Read the model definition and answer for the solid it produces. Units are mm, in the model's axes. Coordinates: 2 decimals unless noted, no trailing zeros. Loops run counter-clockwise (first coordinate to the right, second up) from the corner with the lowest first, then second, coordinate; pieces in that order, holes last.
Q1. Section D-D (y = 65.5) is taken. Give the vertices of the cut face in (x, z), then the cut area to 3 significant figures.
Q2. Section A-A (y = 105) is taken. Give the vertices of the cut face in (x, z).
Q3. Section B-B (x = -461) is taken. Give the vertices of the cut face in (y, z), then the cut area to 4 significant figures.
Q4. Section C-C (z = 2) is taken. Count the separate pieces of the cut face and the enclosed holes in it, then the cut area to 3 significant figures.
Q5. Flat-ended cylindrical pins translate along their axes: P1, Ø1.5, axis at x = -482, z = 3, coming from the +Y side; P2, Ø3, axis at y = 61.5, z = 2, coming from the -X side; P3, Ø1.6, axis at x = -307.5, z = 3, coming from the -Y side. Find the tip coordinate at first contact, or state that the pin passes through.
Q6. The mould has two halves that part along Y. Classify faces 1 (the face through (-176, 106, 3)), 2 (the face through (-171.705, 108.56, 2.712)), 3 (the face through (-304, 76, 0)): pulls with the +Y half, pulls with the -Y half, needs draft (parallel to the pull), parting line crosses it, or undercut.
Q7. Straight lines are drawn through the part: line 1 (X direction, y = 49, z = 3.9); line 2 (X direction, y = 56, z = 0.85); line 3 (X direction, y = 98, z = 4.3). For each, find the intervals that lie inside material, in ascending order.
Autodesk Inventor part; units mm, degrees
ref_plane "YZ Plane" through (0, 0, 0) normal (1, 0, 0) x (0, 1, 0)
ref_plane "XZ Plane" through (0, 0, 0) normal (0, 1, 0) x (-1, 0, 0)
ref_plane "XY Plane" through (0, 0, 0) normal (0, 0, 1) x (1, 0, 0)
sketch "Sketch1" plane through (0, 0, 0) normal (0, 0, 1) x (1, 0, 0)
  line L0 (-280, 0) -> (-280, 5.5)
  line L1 (-280, 5.5) -> (-320, 5.5)
  line L2 (-320, 5.5) -> (-320, 0)
  line L3 (-80, 0) -> (-80, 5.5)
  line L4 (-80, 5.5) -> (-120, 5.5)
  line L5 (-120, 5.5) -> (-120, 0)
  line L6 (-280, 150) -> (-280, 144.5)
  line L7 (-280, 144.5) -> (-320, 144.5)
  line L8 (-320, 144.5) -> (-320, 150)
  line L9 (-80, 150) -> (-80, 144.5)
  line L10 (-80, 144.5) -> (-120, 144.5)
  line L11 (-120, 144.5) -> (-120, 150)
  line L12 (-455, 0) -> (-455, 5.5)
  line L13 (-455, 5.5) -> (-495, 5.5)
  line L14 (-495, 5.5) -> (-495, 0)
  line L15 (-455, 150) -> (-455, 144.5)
  line L16 (-455, 144.5) -> (-495, 144.5)
  line L17 (-495, 144.5) -> (-495, 150)
  line L18 (-600, 55) -> (-594.5, 55)
  line L19 (-594.5, 55) -> (-594.5, 95)
  line L20 (-594.5, 95) -> (-600, 95)
  line L21 (0, 55) -> (-5.5, 55)
  line L22 (-5.5, 55) -> (-5.5, 95)
  line L23 (-5.5, 95) -> (0, 95)
  line L24 (-495, 150) -> (-600, 150)
  line L25 (-455, 150) -> (-320, 150)
  line L26 (-280, 150) -> (-120, 150)
  line L27 (-80, 150) -> (0, 150)
  line L28 (0, 0) -> (-80, 0)
  line L29 (-120, 0) -> (-280, 0)
  line L30 (-320, 0) -> (-455, 0)
  line L31 (-495, 0) -> (-600, 0)
  line L32 (0, 150) -> (0, 95)
  line L33 (0, 55) -> (0, 0)
  line L34 (-600, 150) -> (-600, 95)
  line L35 (-600, 55) -> (-600, 0)
  dimension "d0" = 600
  dimension "d1" = 150
  dimension "d4" = 40
  dimension "d5" = 5.5
  dimension "d8" = 40
  dimension "d9" = 5.5
  dimension "d10" = 40
  dimension "d11" = 5.5
  dimension "d12" = 40
  dimension "d13" = 5.5
  dimension "d14" = 40
  dimension "d15" = 5.5
  dimension "d17" = 5.5
  dimension "d18" = 40
  dimension "d19" = 5.5
  dimension "d23" = 480
extrude "Extrusion1" add sketch "Sketch1" along normal blind 5.5
sketch "Sketch2" plane through (0, 0, 5.5) normal (0, 0, 1) x (1, 0, 0)
  line L0 (-539.343, 36.6) -> (-534.3429, 36.6)
  line L1 (-534.3429, 36.6) -> (-534.3429, 56.6)
  line L2 (-534.3429, 56.6) -> (-539.343, 56.6)
  line L3 (-539.343, 56.6) -> (-539.343, 36.6)
  line L4 (-539.343, 93.3) -> (-534.343, 93.3)
  line L5 (-534.343, 93.3) -> (-534.343, 113.3)
  line L6 (-534.343, 113.3) -> (-539.343, 113.3)
  line L7 (-539.343, 113.3) -> (-539.343, 93.3)
  line L8 (-484.3429, 113.3) -> (-479.3429, 113.3)
  line L9 (-479.3429, 113.3) -> (-479.3429, 93.3)
  line L10 (-479.3429, 93.3) -> (-484.3429, 93.3)
  line L11 (-484.3429, 93.3) -> (-484.3429, 113.3)
  line L12 (-479.3429, 56.6) -> (-484.3429, 56.6)
  line L13 (-484.3429, 56.6) -> (-484.3429, 36.6)
  line L14 (-484.3429, 36.6) -> (-479.3429, 36.6)
  line L15 (-479.3429, 36.6) -> (-479.3429, 56.6)
  line L16 (-600, 150) -> (-600, 95)
  point P0 (0, 0)
  dimension "d26" = 20
  dimension "d27" = 5
  dimension "d28" = 20
  dimension "d29" = 5
  dimension "d30" = 20
  dimension "d33" = 60.657
extrude "Extrusion2" cut sketch "Sketch2" against normal blind 10
sketch "Sketch3" plane through (0, 0, 0) normal (0, 0, -1) x (-1, 0, 0)
  line L0 (181.1029, 114.3822) -> (176.8319, 116.9819)
  line L1 (176.8319, 116.9819) -> (166.433, 99.898)
  line L2 (166.433, 99.898) -> (170.704, 97.2982)
  line L3 (170.704, 97.2982) -> (181.1029, 114.3822)
  point P0 (0, 0)
  dimension "d34" = 5
  dimension "d35" = 20
extrude "Extrusion3" cut sketch "Sketch3" against normal blind 10
properties part number "lado1"
Numbers:
1. outline: (-594.5, 0) - (-5.5, 0) - (-5.5, 5.5) - (-594.5, 5.5) - close
1. area: 3,240 mm2
2. outline: (-600, 0) - (-539.34, 0) - (-539.34, 5.5) - (-600, 5.5) - close; (-534.34, 0) - (-484.34, 0) - (-484.34, 5.5) - (-534.34, 5.5) - close; (-479.34, 0) - (-175.39, 0) - (-175.39, 5.5) - (-479.34, 5.5) - close; (-169.54, 0) - (0, 0) - (0, 5.5) - (-169.54, 5.5) - close
3. outline: (5.5, 0) - (144.5, 0) - (144.5, 5.5) - (5.5, 5.5) - close
3. area: 764.5 mm2
4. separate pieces: 1
4. enclosed holes: 5
4. area: 87,700 mm2
5. P1: stops at y = 144.5
5. P2: stops at x = -594.5
5. P3: stops at y = 5.5
6. face 1: undercut
6. face 2: undercut
6. face 3: needs draft
7. line 1: x = -600 to -539.34, -534.34 to -484.34, -479.34 to 0
7. line 2: x = -594.5 to -539.34, -534.34 to -484.34, -479.34 to -5.5
7. line 3: x = -600 to -539.34, -534.34 to -484.34, -479.34 to -171.13, -169.55 to 0
